Build history of the part. All positions in model axes, mm. Face numbers are marked on the shaded views. A direction names the side the tool comes from. Round coordinates to 2 decimals unless told otherwise and drop trailing zeros. Order: outer loops, then holes, each group sorted by start corner. A loop starts at its lowest first (then second) coordinate and runs counter-clockwise, first axis right, second up. Notation, with made-up numbers: M 63.5,76.5 L 101.5,76.5 A32 ccw 101.5,105.5 Z; hole C 86,69 d10. An arc over 180 degrees is marked long. Use CSV: the item, a comma, the result in double quotes.
from build123d import *

# Parameters (mm, degrees)
F0_W     = 12.7
F0_H     = 203.2
F1_DEPTH = 101.6
F2_W     = 3.175
F2_H     = 12.827
F3_DEPTH = 101.6
F4_R     = 3.5687
F5_DEPTH = 9.525
F6_W     = 6.35
F6_H     = 76.2
F7_DEPTH = 101.6
F8_R     = 3.5687
F9_DEPTH = 6.35


with BuildPart() as f1:
    # F0 (on Front) → F1 (new body)
    with BuildSketch(Plane.XZ):
        with Locations((-51.562002, -57.235944)):
            Rectangle(F0_W, F0_H)
    extrude(amount=F1_DEPTH)

    # F2 (on face) → F3 (cut, through all)
    with BuildSketch(Plane.XZ.offset(101.6)):
        with Locations((-46.799502, -139.722444)):
            Rectangle(F2_W, F2_H)
    extrude(amount=-F3_DEPTH, mode=Mode.SUBTRACT)

    # F4 (on face) → F5 (cut, through all)
    with BuildSketch(Plane.YZ.offset(-48.387002)):
        with Locations((-82.55, -139.722444)):
            Circle(F4_R)
        with Locations((-19.05, -139.722444)):
            Circle(F4_R)
    extrude(amount=-F5_DEPTH, mode=Mode.SUBTRACT)

    # F6 (on face) → F7 (cut, through all)
    with BuildSketch(Plane.XZ.offset(101.6)):
        with Locations((-48.387002, -6.435944)):
            Rectangle(F6_W, F6_H)
    extrude(amount=-F7_DEPTH, mode=Mode.SUBTRACT)

    # F8 (on face) → F9 (cut, through all)
    with BuildSketch(Plane(origin=(-57.912002, 0, 0), x_dir=(0, -1, 0), z_dir=(-1, 0, 0))):
        with Locations((25.4, 18.964056)):
            Circle(F8_R)
        with Locations((25.4, -31.835944)):
            Circle(F8_R)
    extrude(amount=-F9_DEPTH, mode=Mode.SUBTRACT)


solid = f1.part
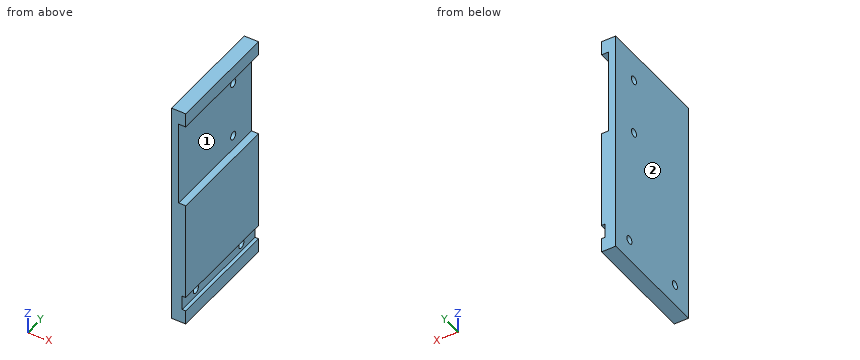
(1) Drop flat-ended pins along their axis: pin 1 (1 mm diameter, centred on y = -14, z = -6.5, fed in from +X); pin 2 (5.5 mm diameter, centred on y = -25.4, z = -31.84, fed in from -X); pin 3 (11.5 mm diameter, centred on y = -19.05, z = -139.72, fed in from +X). Give the stop position or say it passes through.
Answer block:
pin 1,"stops at x = -51.56"
pin 2,"passes through"
pin 3,"stops at x = -48.39"
(2) Wall check: line 1 (Z direction, x = -46, y = -7); line 2 (Z direction, x = -55.75, y = -25.4); line 3 (Z direction, x = -52.25, y = -82.55). Give the ranges that are in metal, low to high. Write a range as from..to.
Answer block:
line 1,"z = -158.84..-146.14, -133.31..-44.54, 31.66..44.36"
line 2,"z = -158.84..-35.4, -28.27..15.4, 22.53..44.36"
line 3,"z = -158.84..-143.29, -136.15..44.36"
(3) Cut at A-A, the plane y = -82.55. Give the cut face in (x, z), and give its area (3 significant figures).
Answer block:
outline,"M -57.91,-158.84 L -45.21,-158.84 L -45.21,-146.14 L -48.39,-146.14 L -48.39,-143.29 L -57.91,-143.29 Z; M -57.91,-136.15 L -48.39,-136.15 L -48.39,-133.31 L -45.21,-133.31 L -45.21,-44.54 L -51.56,-44.54 L -51.56,31.66 L -45.21,31.66 L -45.21,44.36 L -57.91,44.36 Z"
area,"1,990 mm²"
(4) Tool access for the marked faces 1 and 2: list every direction of +Z, -Z, +X, -X, +Y, -Y with a clear straight run to the whole face (end or side of a thin tool).
Answer block:
face 1,"+X, +Y, -Y"
face 2,"+Z, -Z, -X, +Y, -Y"
(5) Cut at D-D, the plane y = -55.5. Give the cut face in (x, z).
Answer block:
outline,"M -57.91,-158.84 L -45.21,-158.84 L -45.21,-146.14 L -48.39,-146.14 L -48.39,-133.31 L -45.21,-133.31 L -45.21,-44.54 L -51.56,-44.54 L -51.56,31.66 L -45.21,31.66 L -45.21,44.36 L -57.91,44.36 Z"
(6) Cut at B-B, the plane y = -25.4. Give the cut face in (x, z), and give its area (3 significant figures).
Answer block:
outline,"M -57.91,-158.84 L -45.21,-158.84 L -45.21,-146.14 L -48.39,-146.14 L -48.39,-133.31 L -45.21,-133.31 L -45.21,-44.54 L -51.56,-44.54 L -51.56,-35.4 L -57.91,-35.4 Z; M -57.91,-28.27 L -51.56,-28.27 L -51.56,15.4 L -57.91,15.4 Z; M -57.91,22.53 L -51.56,22.53 L -51.56,31.66 L -45.21,31.66 L -45.21,44.36 L -57.91,44.36 Z"
area,"1,970 mm²"
(7) Cut at C-C, the plane z = -25. Give the cut face in (x, y), and give its area (3 significant figures).
Answer block:
outline,"M -57.91,-101.6 L -51.56,-101.6 L -51.56,0 L -57.91,0 Z"
area,"645 mm²"
